Autodesk Inventor part; units mm, degrees
ref_plane "Work Plane1" through (0, 69.14, 0) normal (0, 1, 0) x (-1, 0, 0)
ref_plane "Work Plane2" through (0, 0, 6) normal (0, 0, 1) x (1, 0, 0)
ref_plane "YZ Plane" through (0, 0, 0) normal (1, 0, 0) x (0, 1, 0)
sketch "Sketch1" plane through (0, 0, 0) normal (0, 1, 0) x (-1, 0, 0)
  circle A0 centre (0, 0) radius 6
  dimension "d10" = 12
extrude "Extrusion1" add sketch "Sketch1" along normal blind 24.64
sketch "Sketch2" plane through (0, 24.64, 0) normal (0, 1, 0) x (1, 0, 0)
  line L0 (0, 0) -> (9.4, 0) construction
  line L1 (9.4, 0) -> (9.4, -9.4) construction
  line L2 (9.4, -9.4) -> (9.4, 9.4) construction
  line L3 (9.4, 9.4) -> (-7.1118, 9.4) construction
  line L4 (-7.1118, -9.4) -> (25.9118, -9.4)
  line L5 (-7.1118, 9.4) -> (25.9118, 9.4)
  arc A0 (-7.1118, 9.4) -> (-7.1118, -9.4) centre (9.4, 0) ccw
  arc A1 (25.9118, -9.4) -> (25.9118, 9.4) centre (9.4, 0) ccw
  dimension "d3" = 9.4
  dimension "d5" = 9.4
  dimension "d6" = 18.8
extrude "Extrusion2" add sketch "Sketch2" along normal blind 6.35
sketch "Sketch3" plane through (0, 30.99, 0) normal (0, 1, 0) x (1, 0, 0)
  arc A0 (25.9118, -9.4) -> (25.9118, 9.4) centre (9.4, 0) ccw construction
  line L0 (28.4, 0) -> (-9.6, 0) construction
  arc A1 (-7.1118, 9.4) -> (-7.1118, -9.4) centre (9.4, 0) ccw construction
  line L1 (9.4, 0) -> (18.8, 0) construction
  circle A2 centre (18.8, 0) radius 6
  point P0 (0, 0)
  dimension "d9" = 9.4
  dimension "d11" = 12
extrude "Extrusion3" add sketch "Sketch3" along normal blind 8.3
sketch "Sketch4" plane through (18.8, 39.29, 0) normal (0, 1, 0) x (1, 0, 0)
  line L0 (-18.8, 0) -> (-9.4, 0) construction
  line L1 (-25.9118, -9.4) -> (7.1118, -9.4)
  arc A0 (7.1118, -9.4) -> (7.1118, 9.4) centre (-9.4, 0) ccw
  line L2 (-25.9118, -9.4) -> (7.1118, -9.4)
  arc A1 (-25.9118, 9.4) -> (-25.9118, -9.4) centre (-9.4, 0) ccw
  line L3 (-25.9118, 9.4) -> (7.1118, 9.4)
  arc A2 (-25.9118, 9.4) -> (-25.9118, -9.4) centre (-8.6906, 0) ccw
  arc A3 (7.1118, -9.4) -> (7.1118, 9.4) centre (-9.4, 0) ccw
extrude "Extrusion4" add sketch "Sketch4" along normal blind 6.35
sketch "Sketch5" plane through (18.8, 45.64, 0) normal (0, 1, 0) x (1, 0, 0)
  circle A0 centre (-18.8, 0) radius 6
extrude "Extrusion5" add sketch "Sketch5" along normal blind 47
ref_plane "Work Plane1" through (0, 69.14, 0) normal (0, 1, 0) x (-1, 0, 0)
mirror "Mirror1" about plane through (0, 69.14, 0) normal (0, 1, 0) of "Extrusion4", "Extrusion3", "Extrusion2"
sketch "Sketch6" plane through (-7.1118, 113.64, -9.4) normal (0, 1, 0) x (1, 0, 0)
  circle A0 centre (7.1118, -9.4) radius 6
extrude "Extrusion6" add sketch "Sketch6" along normal blind 21.59
sketch "Sketch7" plane through (0, 0, 0) normal (0, 0, 1) x (1, 0, 0)
  line L0 (-6, 0) -> (6, 0) construction
  line L1 (-6, 0) -> (-6, 3.1) construction
  line L2 (-6, 0) -> (-6, 24.64) construction
  line L3 (-6, 3.1) -> (-6, 13.9633) construction
  line L4 (-6, 6.3213) -> (-6.1058, 6.6118) construction
  line L5 (-6, 6.3213) -> (-6, 12.9578) construction
  line L6 (-4, 3.1) -> (-6.1349, 7.8288)
  line L7 (-4, 3.1) -> (-2, 3.1) construction
  line L8 (-4, 3.1) -> (-6, 2.1971)
  line L9 (-6, 2.1971) -> (-6.1349, 7.8288)
  point P0 (0, 0)
extrude "Extrusion7" cut sketch "Sketch7" along normal through all both and the other way through all
ref_plane "Work Plane2" through (0, 0, 6) normal (0, 0, 1) x (1, 0, 0)
sketch "Sketch8" plane through (0, 0, 6) normal (0, 0, 1) x (1, 0, 0)
  line L0 (6, 135.23) -> (-6, 135.23) construction
  line L1 (0, 135.23) -> (0, 122.73) construction
  line L2 (0, 122.73) -> (0, 119.73) construction
  line L3 (2, 116.73) -> (-2, 116.73)
  line L4 (-2, 116.73) -> (-2, 122.73)
  line L5 (-2, 122.73) -> (2, 122.73)
  line L6 (2, 122.73) -> (2, 116.73)
  line L7 (2, 116.73) -> (-2, 122.73) construction
  line L8 (-2, 116.73) -> (2, 122.73) construction
  point P0 (0, 0)
  dimension "d29" = 12.5
  dimension "d30" = 3
  dimension "d31" = 4
extrude "Extrusion8" cut sketch "Sketch8" against normal blind 0.5
properties part number "Albero a gomito"
Work out the finished part from the listing and answer in its coordinate system (mm). A direction names the side the tool comes from. Give positions to 0.01 mm unless a question says otherwise; leave off trailing zeros. Write each loop counter-clockwise with the first axis right and the second up, starting at its lowest first coordinate (ties: lowest second). Pieces come first, ordered by that corner, then holes. Notation, with made-up numbers: (-30.5, 87.25) -> (2.5, 87.25) arc R18 ccw to (2.5, 106.25) -> close; hole circle Ø8 at (-2, 33). An arc over 180 degrees is marked (long way). Write item = value, one per line.
Q1. Section C-C on z = -7.75 is taken. Determine the outline of the cut face in (x, y), and give its area (3 significant figures).
Computed values:
outline = (-7.95, 24.64) -> (26.75, 24.64) -> (26.75, 30.99) -> (-7.95, 30.99) -> close; (-7.95, 39.29) -> (26.75, 39.29) -> (26.75, 45.64) -> (-7.95, 45.64) -> close; (-7.95, 92.64) -> (26.75, 92.64) -> (26.75, 98.99) -> (-7.95, 98.99) -> close; (-7.95, 107.29) -> (26.75, 107.29) -> (26.75, 113.64) -> (-7.95, 113.64) -> close
area = 881 mm^2
Q2. Section D-D on y = 71 is taken. Determine the outline of the cut face in (x, z).
Computed values:
outline = circle Ø12 at (0, 0)
Q3. Section A-A on x = 0 is taken. State how many separate pieces and enclosed holes the cut face has, and give its area (3 significant figures).
Computed values:
separate_pieces = 3
enclosed_holes = 0
area = 1,590 mm^2
Q4. For a pull along Y with two mould halves and no side action, classify faces 1 (the cylindrical face through (-9.6, 27.8, 0.1)), 2 (the flat face through (0, 135.23, 0)), 3 (the flat face through (13, 45.64, 0)) as pulls with the +Y half, pulls with the -Y half, needs draft (parallel to the pull), parting line crosses it, or undercut.
Computed values:
face_1 = needs draft
face_2 = pulls with the +Y half
face_3 = undercut
Q5. Section B-B on x = 18.8 is taken. Determine the outline of the cut face in (y, z), and give its area (3 significant figures).
Computed values:
outline = (24.64, -9.4) -> (30.99, -9.4) -> (30.99, -6) -> (39.29, -6) -> (39.29, -9.4) -> (45.64, -9.4) -> (45.64, 9.4) -> (39.29, 9.4) -> (39.29, 6) -> (30.99, 6) -> (30.99, 9.4) -> (24.64, 9.4) -> close; (92.64, -9.4) -> (98.99, -9.4) -> (98.99, -6) -> (107.29, -6) -> (107.29, -9.4) -> (113.64, -9.4) -> (113.64, 9.4) -> (107.29, 9.4) -> (107.29, 6) -> (98.99, 6) -> (98.99, 9.4) -> (92.64, 9.4) -> close
area = 677 mm^2
Q6. Consider line 1 along Y through (x, z) = (7, -3.25); line 2 along Y through (x, z) = (14.5, -1); line 3 along X through (y, z) = (128, 0.25). Determine where each line is inside the solid, lowest interval first.
Computed values:
line_1 = 24.64 to 30.99, 39.29 to 45.64, 92.64 to 98.99, 107.29 to 113.64
line_2 = 24.64 to 45.64, 92.64 to 113.64
line_3 = -5.99 to 5.99
Q7. Flat-ended cylindrical pins translate along their axes: pin 1 Ø3 at (x, y) = (6.5, 80) entering from +Z; pin 2 Ø6 at (y, z) = (62.5, 3) entering from +X; pin 3 Ø9.5 at (x, z) = (16.5, 1.5) entering from +Y. Find the tip coordinate at first contact, or state that the pin passes through.
Computed values:
pin_1 = 3.32
pin_2 = 6
pin_3 = 113.64
Q8. A tool of negligible diameter and unlimited length cuts with its end or side. For faces 4 (the cylindrical face through (-1.301, 124.284, -5.857)), 5 (the cylindrical face through (28.4, 95.9, 0.1)), from which of +Z, -Z, +X, -X, +Y, -Y can it reach the whole face along a straight path? Write none if from no direction.
Computed values:
face_4 = +Y
face_5 = +X, +Y, -Y
